Design review of the part built by this model. Coordinates are the model's own, in mm. A direction names the side the tool comes from. Coordinates: 2 decimals unless noted, no trailing zeros. Write each loop counter-clockwise with the first axis right and the second up, starting at its lowest first coordinate (ties: lowest second). Pieces come first, ordered by that corner, then holes. Notation, with made-up numbers: (63.5, 31) -> (87.5, 31) arc R22 ccw to (87.5, 41) -> close; hole circle Ø8 at (-14, -6.75). An arc over 180 degrees is marked (long way). Return JSON: item names as keys, results as strings. Group by question number.
from build123d import *

# Parameters (mm, degrees)
BOSS_EXTRUDE1_DEPTH     = 30
FILLET1_R               = 10
SKETCH2_R               = 2
CUT_EXTRUDE1_DEPTH      = 1
CUT_EXTRUDE1_DEPTH_BACK = 257


with BuildPart() as part:
    # Sketch1 → Boss-Extrude1 (new body)
    with BuildSketch(Plane.XY):
        Polygon((128, -127), (125, -127), (125, -108.051382857), (41.057072577, -3), (-41.057072577, -3), (-125, -108.051382857), (-125, -127), (-128, -127), (-128, -107), (-42.5, 0), (42.5, 0), (128, -107), align=None)
    extrude(amount=BOSS_EXTRUDE1_DEPTH)

    # Fillet1
    fillet1_edges = [part.edges().sort_by_distance(p)[0] for p in [
        (125, -108.051382857, 15),
        (41.057072577, -3, 15),
        (-41.057072577, -3, 15),
        (-125, -108.051382857, 15),
        (-128, -107, 15),
        (-42.5, 0, 15),
        (42.5, 0, 15),
        (128, -107, 15),
    ]]
    fillet(fillet1_edges, radius=FILLET1_R)

    # Sketch2 → Cut-Extrude1 (cut, two sides)
    with BuildSketch(Plane(origin=(128, 0, 0), x_dir=(0, 0, -1), z_dir=(1, 0, 0))) as cut_extrude1_sk:
        with Locations((-15, -117)):
            Circle(SKETCH2_R)
    extrude(amount=CUT_EXTRUDE1_DEPTH, mode=Mode.SUBTRACT)
    extrude(cut_extrude1_sk.sketch, amount=-CUT_EXTRUDE1_DEPTH_BACK, mode=Mode.SUBTRACT)


solid = part.part
Q1. We need section A-A on z = 23. Write out the cut boundary in (x, y).
Q2. For P1, Ø3, axis at y = -35, z = 12, coming from the -X side; P2, Ø9, axis at x = 6.5, z = 22, coming from the -Y side; P3, Ø2, axis at y = -65, z = 24.5, coming from the +X side, all flat-tipped, find the tip position at first contact; note any pin that passes through.
Q3. The part is to be moulded in two halves that separate along X. For faces 3 (the cylindrical face through (-42.081, -1.016, 15.21)), 4 (the flat face through (1, -2, 30)), 5 (the cylindrical face through (40.638, -4.016, 15.21)), say which applies: +X half, -X half, draft (parallel to the pull), parting line (faces both ways), or undercut.
Q4. For faces 1 (the flat face through (-82.885, -55.346, 14.79)), 2 (the flat face through (-1, 0, 15)), list the 3-axis set-ups (+Z, -Z, +X, -X, +Y, -Y) from which the entire face can be reached by the end or side of a thin tool; tool diameter is ignored.
Q5. We need section D-D on x = -89. Write out the cut boundary in (y, z), plus the area to 3 significant figures.
Q6. Wall thickness on L1, parallel to Y at x = 126.55, z = 15; L2, parallel to Y at x = 2, z = 27.25; L3, parallel to X at y = -99, z = 20.75: over which ranges is each line inside the solid? List them lowest first.
Q7. We need section B-B on y = -52.5. Write out the cut boundary in (x, z).
Q8. We need section C-C on x = -31. Write out the cut boundary in (y, z), plus the area to 3 significant figures.
Findings below:
{
 "1": {"outline": "(-128, -127) -> (-125, -127) -> (-125, -111.56) arc R10 cw to (-122.81, -105.31) -> (-44.06, -6.76) arc R10 cw to (-36.25, -3) -> (36.25, -3) arc R10 cw to (44.06, -6.76) -> (122.81, -105.31) arc R10 cw to (125, -111.56) -> (125, -127) -> (128, -127) -> (128, -110.5) arc R10 ccw to (125.81, -104.26) -> (45.5, -3.76) arc R10 ccw to (37.69, 0) -> (-37.69, 0) arc R10 ccw to (-45.5, -3.76) -> (-125.81, -104.26) arc R10 ccw to (-128, -110.5) -> close"},
 "2": {"P1": "stops at x = -71.67", "P2": "stops at y = -3", "P3": "stops at x = 95.24"},
 "3": {"face 3": "-X half", "face 4": "draft", "face 5": "undercut"},
 "4": {"face 1": "+Z, -Z, -Y", "face 2": "+Z, -Z, +X, -X, +Y"},
 "5": {"outline": "(-63, 0) -> (-58.19, 0) -> (-58.19, 30) -> (-63, 30) -> close", "area": "144 mm^2"},
 "6": {"L1": "y = -127 to -119, -115 to -105.32", "L2": "y = -3 to 0", "L3": "x = -121.61 to -117.77, 117.77 to 121.61"},
 "7": {"outline": "(-84.45, 0) -> (-80.61, 0) -> (-80.61, 30) -> (-84.45, 30) -> close; (80.61, 0) -> (84.45, 0) -> (84.45, 30) -> (80.61, 30) -> close"},
 "8": {"outline": "(-3, 0) -> (0, 0) -> (0, 30) -> (-3, 30) -> close", "area": "90.0 mm^2"}
}
